Read the model definition and answer for the solid it produces. Units are mm, in the model's axes. Face numbers are marked on the shaded views. Coordinates: 2 decimals unless noted, no trailing zeros. Write each loop counter-clockwise with the first axis right and the second up, starting at its lowest first coordinate (ties: lowest second). Pieces come first, ordered by that corner, then holes. Notation, with made-up numbers: (87, 47.5) - (145, 47.5) arc R10 cw to (145, 51.5) - close; hole circle Ø10 at (-18.75, -25.5). An arc over 180 degrees is marked (long way). Return JSON: item names as keys, results as strings.
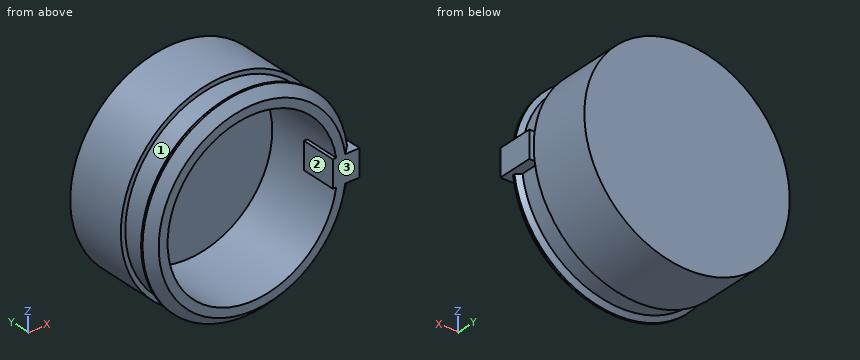
```python
from build123d import *

# Parameters (mm, degrees)
F0_R        = 11.5
F0_R_2      = 9.5
F1_DEPTH    = 7
F2_DEPTH    = 2
F3_R        = 11
F3_R_2      = 9.5
F4_DEPTH    = 2
F5_R        = 11.5
F5_R_2      = 11
F5_R_3      = 9.5
F6_DEPTH    = 2
F7_S5_R     = 11
F7_T6_DEPTH = 18
F8_SIZE     = 1
F9_W        = 3
F9_H        = 3
F10_DEPTH   = 4


# Not quite as in the source:
# - a fillet or chamfer that OpenCascade refuses, or shapes differently, is made with other operations: its cross-section is extruded or revolved along the edge and cut away or added


with BuildPart() as f1:
    # F0 (on Front) → F1 (new body)
    with BuildSketch(Plane.XZ):
        Circle(F0_R)
        Circle(F0_R_2, mode=Mode.SUBTRACT)
    extrude(amount=F1_DEPTH)

    # F0 (on Front) → F2 (join)
    with BuildSketch(Plane.XZ):
        Circle(F0_R_2)
    extrude(amount=F2_DEPTH)

    # F3 (on face) → F4 (join)
    with BuildSketch(Plane.XZ.offset(7)):
        Circle(F3_R)
        Circle(F3_R_2, mode=Mode.SUBTRACT)
    extrude(amount=F4_DEPTH)

    # F5 (on face) → F6 (join)
    with BuildSketch(Plane.XZ.offset(9)):
        Circle(F5_R)
        Circle(F5_R_2, mode=Mode.SUBTRACT)
        Circle(F5_R_2)
        Circle(F5_R_3, mode=Mode.SUBTRACT)
    extrude(amount=F6_DEPTH)

    # F7: chamfer of 0.8 on 1 edges, made by hand


with BuildPart() as f7_tool2:
    # F7_s3 → F7_t4 (revolve)
    with BuildSketch(Plane.XY):
        Polygon((10.7, -9), (11.5, -9.8), (11.5, -9), align=None)
    revolve(axis=Axis((0, -9, 0), (0, -1, 0)))

    # F7_s5 → F7_t6 (cut, symmetric)
    with BuildSketch(Plane.XZ.offset(9.4)):
        Circle(F7_S5_R)
    extrude(amount=F7_T6_DEPTH, both=True, mode=Mode.SUBTRACT)


with BuildPart() as f1_1:
    add(f1.part)

    # F7_t1: cut F7_tool2
    add(f7_tool2.part, mode=Mode.SUBTRACT)

    # F8
    f8_edges = [f1_1.edges().sort_by_distance(p)[0] for p in [
        (-11.5, -11, 0),
    ]]
    chamfer(f8_edges, length=F8_SIZE)

    # F9 (on face) → F10 (join)
    with BuildSketch(Plane.XZ.offset(11)):
        with Locations((10.5, 0)):
            Rectangle(F9_W, F9_H)
    extrude(amount=-F10_DEPTH)


solid = f1_1.part
```
(1) A cutting plane is placed at D-D (y = -1.5). Determine the outline of the cut face in (x, z).
Answer:
{"outline": "circle Ø23 at (0, 0)"}
(2) A cutting plane is placed at B-B (z = 0). Determine the outline of the cut face in (x, y), and give its area (3 significant figures).
Answer:
{"outline": "(-11.5, -10) - (-10.5, -11) - (-9.5, -11) - (-9.5, -2) - (9.5, -2) - (9.5, -7) - (9, -7) - (9, -11) - (12, -11) - (12, -7) - (11.5, -7) - (11.5, 0) - (-11.5, 0) - (-11.5, -7) - (-11, -7) - (-11, -9.3) - (-11.5, -9.8) - close", "area": "84.2 mm²"}
(3) Straight lines are drawn through the part: line 1 (X direction, y = -5.5, z = 0); line 2 (X direction, y = -7.5, z = 0.25). For each, find the intervals that lie inside material, in ascending order. Write a range as from..to.
Answer:
{"line 1": "-11.5..-9.5, 9.5..11.5", "line 2": "-11..-9.5, 9..12"}
(4) A cutting plane is placed at C-C (x = 0). Determine the outline of the cut face in (y, z).
Answer:
{"outline": "(-11, -10.5) - (-10, -11.5) - (-9.8, -11.5) - (-9.3, -11) - (-7, -11) - (-7, -11.5) - (0, -11.5) - (0, 11.5) - (-7, 11.5) - (-7, 11) - (-9.3, 11) - (-9.8, 11.5) - (-10, 11.5) - (-11, 10.5) - (-11, 9.5) - (-2, 9.5) - (-2, -9.5) - (-11, -9.5) - close"}
(5) Determine the mould class of the marked faces 1, 2 and 3 for opening direction Y: +Y half, -Y half, draft (parallel to the pull), parting line (faces both ways), or undercut.
Answer:
{"face 1": "undercut", "face 2": "draft", "face 3": "-Y half"}
(6) A cutting plane is placed at A-A (y = -8.25). Determine the outline of the cut face in (x, z).
Answer:
{"outline": "(10.9, -1.5) - (12, -1.5) - (12, 1.5) - (10.9, 1.5) arc R11 ccw (long way) to start; hole (9, -1.5) - (9, 1.5) - (9.38, 1.5) arc R9.5 ccw (long way) to (9.38, -1.5) - close"}
(7) Flat-ended cylindrical pins translate along their axes: P1, Ø2, axis at y = -6, z = -3, coming from the -X side; P2, Ø5, axis at x = 3, y = -7, coming from the +Z side; P3, Ø5, axis at x = 5.5, y = -6.5, coming from the -Z side. Find the tip coordinate at first contact, or state that the pin passes through.
Answer:
{"P1": "x = -11.32", "P2": "z = 11.49", "P3": "z = -11.1"}
